```python
from build123d import *

# Parameters (mm, degrees)
SKETCH1_W               = 42.1
SKETCH1_H               = 50
BOSS_EXTRUDE1_DEPTH     = 17.1
SKETCH2_R               = 2.6
CUT_EXTRUDE1_DEPTH      = 37.885125728
MIRROR3_COPY_1_SKETCH_R = 2.6
MIRROR3_COPY_1_DEPTH    = 37.885125728
SKETCH3_R               = 4.5
CUT_EXTRUDE2_DEPTH      = 57.881565555
SKETCH4_R               = 8
CUT_EXTRUDE3_DEPTH      = 10
FILLET1_R               = 1


with BuildPart() as part:
    # Sketch1 → Boss-Extrude1 (new body)
    with BuildSketch(Plane(origin=(0, 0, 0), x_dir=(1, 0, 0), z_dir=(0, 1, 0))):
        Rectangle(SKETCH1_W, SKETCH1_H)
    extrude(amount=BOSS_EXTRUDE1_DEPTH)

    # Sketch2 → Cut-Extrude1 (cut, through all)
    with BuildSketch(Plane(origin=(0, 17.1, 0), x_dir=(1, 0, 0), z_dir=(0, 1, 0))):
        with Locations(Location((-16, -20, 0), (0, 0, 270))):
            Circle(SKETCH2_R)
    cut_extrude1 = extrude(amount=-CUT_EXTRUDE1_DEPTH, mode=Mode.SUBTRACT)

    # Mirror2: Cut-Extrude1 across plane
    add(cut_extrude1.mirror(Plane.XY), mode=Mode.SUBTRACT)

    # Mirror3: Cut-Extrude1 across plane
    add(cut_extrude1.mirror(Plane(origin=(0, 0, 0), x_dir=(0, 0, 1), z_dir=(1, 0, 0))), mode=Mode.SUBTRACT)

    # Mirror3 copy 1 sketch → Mirror3 copy 1 (cut, through all)
    with BuildSketch(Plane(origin=(0, 17.1, 0), x_dir=(-1, 0, 0), z_dir=(0, 1, 0))):
        with Locations(Location((-16, -20, 0), (0, 0, 270))):
            Circle(MIRROR3_COPY_1_SKETCH_R)
    extrude(amount=-MIRROR3_COPY_1_DEPTH, mode=Mode.SUBTRACT)

    # Sketch3 → Cut-Extrude2 (cut, through all)
    with BuildSketch(Plane.XY.offset(25)):
        Circle(SKETCH3_R)
    extrude(amount=-CUT_EXTRUDE2_DEPTH, mode=Mode.SUBTRACT)

    # Sketch4 → Cut-Extrude3 (cut)
    with BuildSketch(Plane.XY.offset(25)):
        Circle(SKETCH4_R)
    extrude(amount=-CUT_EXTRUDE3_DEPTH, mode=Mode.SUBTRACT)

    # Fillet1
    fillet1_edges = [part.edges().sort_by_distance(p)[0] for p in [
        (-21.05, 17.1, 0),
        (0, 17.1, 25),
        (-12.775, 0, -25),
        (4.5, 0, -5),
        (0, 4.5, -25),
        (21.05, 17.1, 0),
        (-4.5, 0, -5),
        (0, 4.5, 15),
        (14.525, 0, 25),
        (-14.525, 0, 25),
        (8, 0, 20),
        (-8, 0, 20),
        (0, 8, 15),
        (6.25, 0, 15),
        (-6.25, 0, 15),
        (0, 8, 25),
        (-21.05, 0, 0),
        (12.775, 0, -25),
        (21.05, 0, 0),
        (0, 17.1, -25),
        (21.05, 8.55, 25),
        (-21.05, 8.55, 25),
        (-21.05, 8.55, -25),
        (21.05, 8.55, -25),
    ]]
    fillet(fillet1_edges, radius=FILLET1_R)


solid = part.part
```
Model file for the job. Use its own axes, mm. Round coordinates to 2 decimals unless told otherwise and drop trailing zeros. Loops run counter-clockwise (first coordinate to the right, second up) from the corner with the lowest first, then second, coordinate; pieces in that order, holes last. Notation, with made-up numbers: M 79.25,-20.75 L 86.25,-20.75 A32 ccw 86.25,14.25 Z; hole C -25,-14 d6. An arc over 180 degrees is marked long. Put each result on its own line as item: value. Start each with the question number.
Item 1: Cut at C-C (y = 13). List the corners of the cut face in (x, z).
Item 2: Cut at D-D (z = 7.5). List the corners of the cut face in (x, y) (3 decimals), then the cut area to 3 significant figures.
Item 3: Drop flat-ended pins along their axis: P1, Ø4, axis at x = 4, y = 3.5, coming from the +Z side; P2, Ø3, axis at x = 2, y = 5, coming from the +Z side. Give the stop position or say it passes through.
Item 4: Cut at A-A (x = 16). List the corners of the cut face in (y, z), then the cut area to 3 significant figures.
Item 5: Cut at B-B (z = -20). List the corners of the cut face in (x, y) (3 decimals), then the cut area to 3 significant figures.
Item 6: Mould opens along Z. For faces 1 (the face through (0, 6, 15)), 2 (the face through (0, 8, 20)), 3 (the face through (-17, 8.7, 22.4)) say: released by +Z, released by -Z, zero draft, split by the parting line, or undercut.
Item 7: Drill centre lines: line 1 along Z through (x, y) = (16, 8.5); line 2 along X through (y, z) = (12.5, 20); line 3 along X through (y, z) = (4.5, 20). Where is each one in solid material? Low to high.
Answer block:
1. outline: M -21.05,-24 A1 ccw -20.05,-25 L 20.05,-25 A1 ccw 21.05,-24 L 21.05,24 A1 ccw 20.05,25 L -20.05,25 A1 ccw -21.05,24 Z; hole C -16,-20 d5.2; hole C -16,20 d5.2; hole C 16,-20 d5.2; hole C 16,20 d5.2
2. outline: M -21.05,1 A1 ccw -20.05,0 L -5.408,0 A1 ccw -4.425,0.818 A4.5 cw 4.425,0.818 A1 ccw 5.408,0 L 20.05,0 A1 ccw 21.05,1 L 21.05,16.1 A1 ccw 20.05,17.1 L -20.05,17.1 A1 ccw -21.05,16.1 Z
2. area: 687 mm2
3. P1: z = 15.05
3. P2: z = 15
4. outline: M 0,-24 A1 ccw 1,-25 L 16.1,-25 A1 ccw 17.1,-24 L 17.1,-22.6 L 0,-22.6 Z; M 0,-17.4 L 17.1,-17.4 L 17.1,17.4 L 0,17.4 Z; M 0,22.6 L 17.1,22.6 L 17.1,24 A1 ccw 16.1,25 L 1,25 A1 ccw 0,24 Z
4. area: 676 mm2
5. outline: M -21.05,1 A1 ccw -20.05,0 L -18.6,0 L -18.6,17.1 L -20.05,17.1 A1 ccw -21.05,16.1 Z; M -13.4,0 L -5.408,0 A1 ccw -4.425,0.818 A4.5 cw 4.425,0.818 A1 ccw 5.408,0 L 13.4,0 L 13.4,17.1 L -13.4,17.1 Z; M 18.6,0 L 20.05,0 A1 ccw 21.05,1 L 21.05,16.1 A1 ccw 20.05,17.1 L 18.6,17.1 Z
5. area: 509 mm2
6. face 1: released by +Z
6. face 2: zero draft
6. face 3: undercut
7. line 1: -25 to -22.6, -17.4 to 17.4, 22.6 to 25
7. line 2: -21.05 to -18.6, -13.4 to 13.4, 18.6 to 21.05
7. line 3: -21.05 to -18.6, -13.4 to -6.61, 6.61 to 13.4, 18.6 to 21.05
